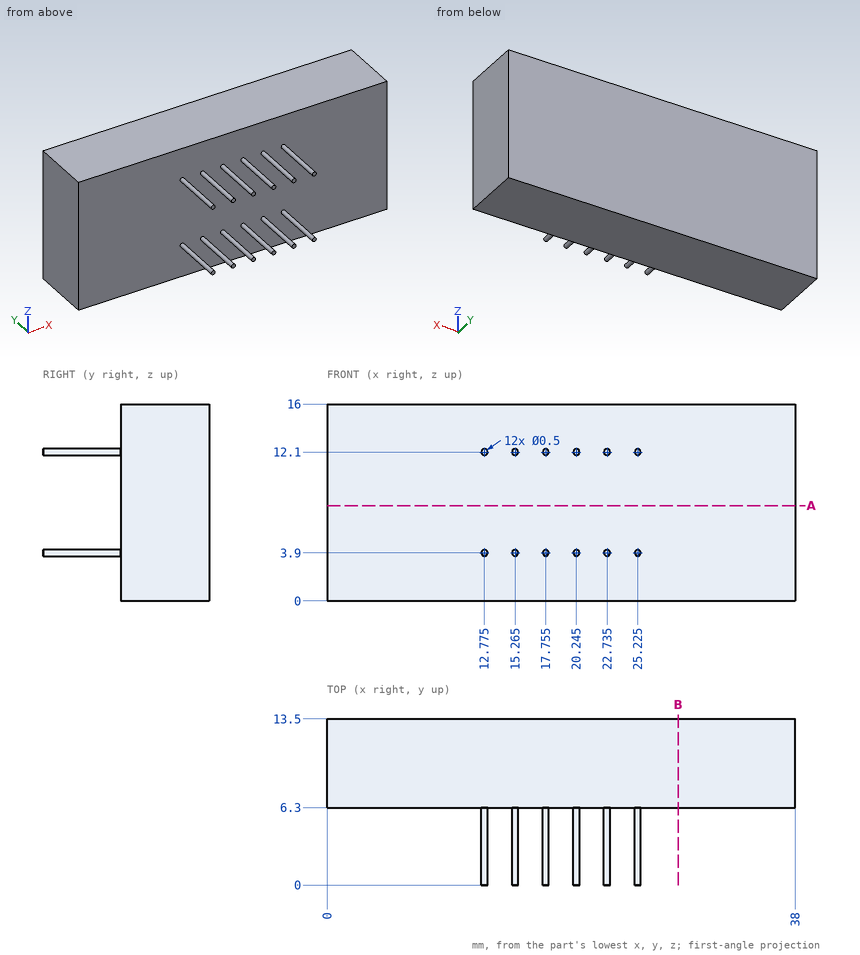
Here's the drawing with two shaded views (mm, measured from the low corner). I have some questions. Coordinates: 2 decimals unless noted, no trailing zeros. Loops run counter-clockwise (first coordinate to the right, second up) from the corner with the lowest first, then second, coordinate; pieces in that order, holes last. Notation, with made-up numbers: M 26,68.25 L 52,68.25 A32 ccw 52,104.25 Z; hole C -1.75,39.25 d7. An arc over 180 degrees is marked long. Put each result on its own line as item: value. Start each with the question number.
(1) Imagine slicing it at A-A on z = 7.75. List the corners of the cut face in (x, y) for me, and give its area (3 significant figures).
(2) Imagine slicing it at B-B on x = 28.5. List the corners of the cut face in (y, z) for me, and give its area (3 significant figures).
(3) I need wall thicknesses on probe 1 along Y at (x, z) = (33, 2.5). Which ranges of the line are inside material? Lowest first, please.
(4) Will these pins go through, and if not, where does the flat tip stop? pin 1 Ø1 at (y, z) = (2.5, 10.5) entering from +X; pin 2 Ø4 at (y, z) = (4, 10.5) entering from -X (1 decimal); pin 3 Ø4 at (y, z) = (9.5, 2.5) entering from -X.
Worked answers:
1. outline: M 0,6.3 L 38,6.3 L 38,13.5 L 0,13.5 Z
1. area: 274 mm2
2. outline: M 6.3,0 L 13.5,0 L 13.5,16 L 6.3,16 Z
2. area: 115 mm2
3. probe 1: y = 6.3 to 13.5
4. pin 1: passes through
4. pin 2: stops at x = 12.5
4. pin 3: stops at x = 0
